Part print with two shaded views. Sizes in mm from the minimum x, y, z corner. A direction names the side the tool comes from. Round coordinates to 2 decimals unless told otherwise and drop trailing zeros. Order: outer loops, then holes, each group sorted by start corner. A loop starts at its lowest first (then second) coordinate and runs counter-clockwise, first axis right, second up. Notation, with made-up numbers: (61, -25.5) - (97, -25.5) arc R26 cw to (97, -2.5) - close; hole circle Ø1 at (49, 38.25). An arc over 180 degrees is marked (long way). Use one line per item in the form item = value.
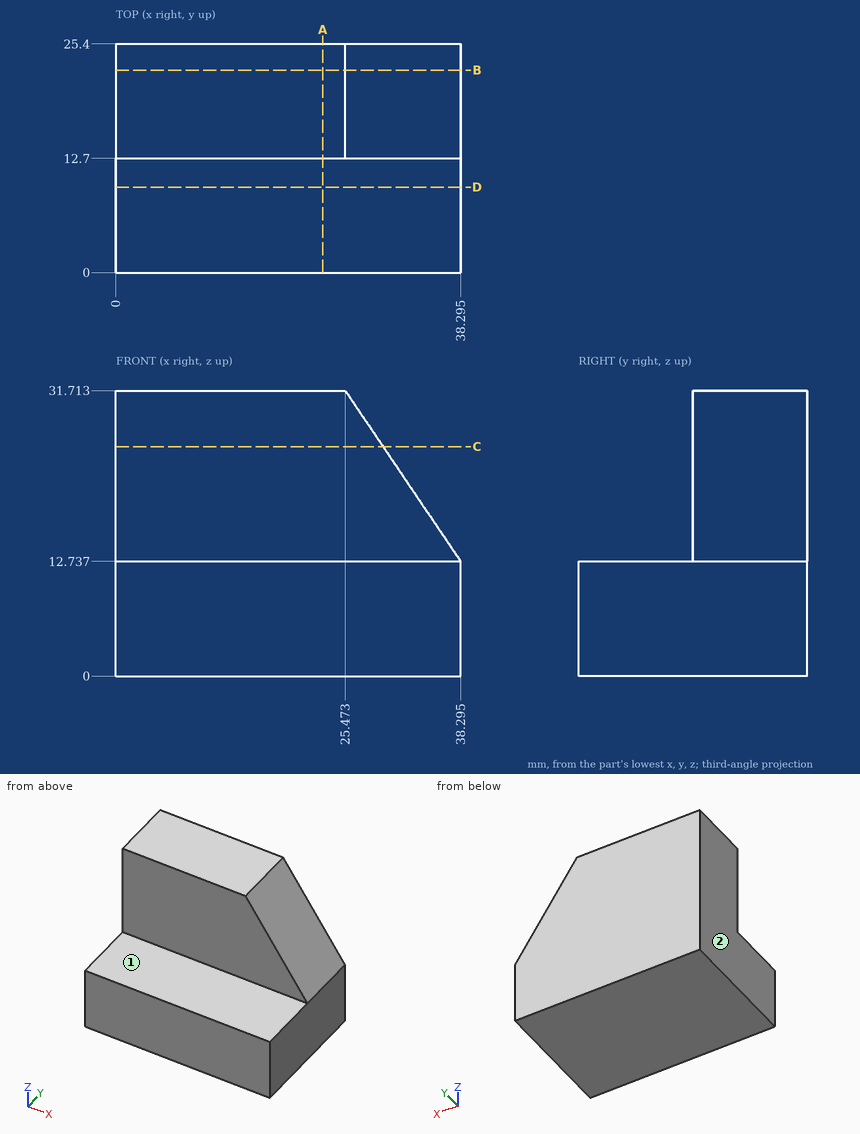
(1) Slice it at A-A on x = 23. Give the cut face in (y, z).
Report:
outline = (0, 0) - (25.4, 0) - (25.4, 31.71) - (12.7, 31.71) - (12.7, 12.74) - (0, 12.74) - close
(2) Slice it at C-C on z = 25.5. Give the cut face in (x, y).
Report:
outline = (0, 12.7) - (29.67, 12.7) - (29.67, 25.4) - (0, 25.4) - close
(3) Probe probe 1 along Z at (x, y) = (19.5, 5.5); probe 2 along Y at (x, z) = (21, 21); probe 3 along X at (y, z) = (14.25, 29) (1 decimal). List the from-to ranges inside material, lowest first. Write a range as [from, to].
Report:
probe_1 = [0, 12.74]
probe_2 = [12.7, 25.4]
probe_3 = [0, 27.3]
(4) Slice it at B-B on y = 22.5. Give the cut face in (x, z) (1 decimal), then the cut area to 3 significant figures.
Report:
outline = (0, 0) - (38.3, 0) - (38.3, 12.7) - (25.5, 31.7) - (0, 31.7) - close
area = 1,090 mm2
(5) Tool access for the marked faces 1 and 2: list every direction of +Z, -Z, +X, -X, +Y, -Y with a clear straight run to the whole face (end or side of a thin tool).
Report:
face_1 = +Z, +X, -X, -Y
face_2 = +Z, -Z, -X, +Y, -Y
(6) Slice it at D-D on y = 9.5. Give the cut face in (x, z) (1 decimal), then the cut area to 3 significant figures.
Report:
outline = (0, 0) - (38.3, 0) - (38.3, 12.7) - (0, 12.7) - close
area = 488 mm2
(7) Pin check, flat tips, straight feed: pin 1 (4 mm diameter, centred on x = 14.5, y = 9.5, fed in from +Z); pin 2 (8 mm diameter, centred on y = 16, z = 23.5, fed in from +X) (1 decimal); pin 3 (1.5 mm diameter, centred on x = 15, z = 19.5, fed in from -Y); pin 4 (1 mm diameter, centred on y = 10, z = 13.5, fed in from +X). Stop position of each tip, or through.
Report:
pin_1 = 12.74
pin_2 = 33.7
pin_3 = 12.7
pin_4 = through
